Geometry check sheet. Reference: the model listing, model coordinates, mm. Coordinates: 2 decimals unless noted, no trailing zeros. Order: outer loops, then holes, each group sorted by start corner. A loop starts at its lowest first (then second) coordinate and runs counter-clockwise, first axis right, second up. Notation, with made-up numbers: (-37.75, 52.5) - (-21.75, 52.5) arc R18 cw to (-21.75, 80.5) - close; hole circle Ø6 at (48.25, 54). An arc over 180 degrees is marked (long way). Put each result on its own line as item: value.
from build123d import *

# Parameters (mm, degrees)
SKETCH_1_W          = 20
SKETCH_1_H          = 20
SKETCH_1_W_2        = 18
SKETCH_1_H_2        = 18
EXTRUDE_1_DEPTH     = 180
SKETCH_2_R          = 1.6
CUT_EXTRUDE_1_DEPTH = 50


with BuildPart() as part:
    # 草图1 → 凸台-拉伸1 (new body)
    with BuildSketch(Plane.XY):
        Rectangle(SKETCH_1_W, SKETCH_1_H)
        Rectangle(SKETCH_1_W_2, SKETCH_1_H_2, mode=Mode.SUBTRACT)
    extrude(amount=EXTRUDE_1_DEPTH)

    # 草图2 → 切除-拉伸1 (cut)
    with BuildSketch(Plane(origin=(0, 10, 0), x_dir=(1, 0, 0), z_dir=(0, 1, 0))):
        with Locations(Location((0, -90, 0), (0, 0, 270))):
            Circle(SKETCH_2_R)
        with Locations(Location((0, -170, 0), (0, 0, 270))):
            Circle(SKETCH_2_R)
        with Locations(Location((0, -10, 0), (0, 0, 270))):
            Circle(SKETCH_2_R)
    extrude(amount=-CUT_EXTRUDE_1_DEPTH, mode=Mode.SUBTRACT)


solid = part.part
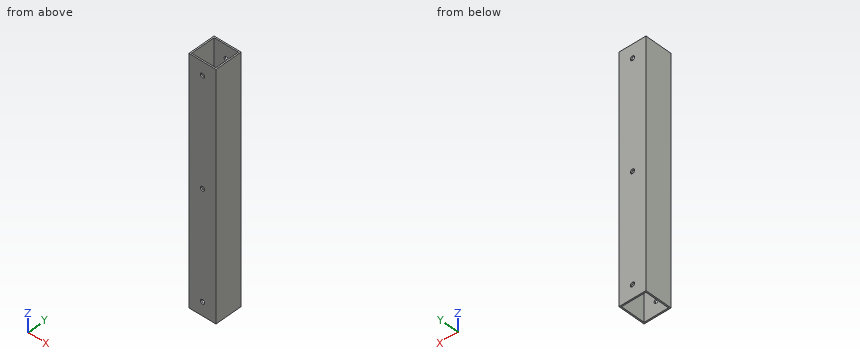
Q1. Section check B-B on z = 90. Record the boundary of the cut face in (x, y).
Answer block:
outline: (-10, -10) - (-1.6, -10) - (-1.6, -9) - (-9, -9) - (-9, 9) - (-1.6, 9) - (-1.6, 10) - (-10, 10) - close; (1.6, -10) - (10, -10) - (10, 10) - (1.6, 10) - (1.6, 9) - (9, 9) - (9, -9) - (1.6, -9) - close
Q2. Thickness scan on L1, parallel to Y at x = 2, z = 122; L2, parallel to X at y = 9.55, z = 90. Record the ranges inside material, lowest first. Write a range as [from, to].
Answer block:
L1: y = [-10, -9], [9, 10]
L2: x = [-10, -1.6], [1.6, 10]
Q3. Section check D-D on x = 0. State how many separate pieces and enclosed holes the cut face has, then the cut area to 3 significant figures.
Answer block:
separate pieces: 8
enclosed holes: 0
area: 341 mm^2
Q4. Section check A-A on x = 7.5. Record the boundary of the cut face in (y, z), then the cut area to 3 significant figures.
Answer block:
outline: (-10, 0) - (-9, 0) - (-9, 180) - (-10, 180) - close; (9, 0) - (10, 0) - (10, 180) - (9, 180) - close
area: 360 mm^2
